Here's how the part is built. I have some questions about the finished solid (model axes, mm). Coordinates: 2 decimals unless noted, no trailing zeros. Write each loop counter-clockwise with the first axis right and the second up, starting at its lowest first coordinate (ties: lowest second). Pieces come first, ordered by that corner, then holes. Notation, with made-up numbers: (-30, 44) -> (15, 44) arc R19 ccw to (15, 79) -> close; hole circle Ø8 at (-38, 3.5). An arc over 180 degrees is marked (long way). Put each result on its own line as item: value. Start each with the question number.
Item 1: I need wall thicknesses on line 1 (X direction, y = -1, z = -1); line 2 (Z direction, x = 2, y = -0.05); line 3 (Z direction, x = -2, y = -0.9). Which ranges of each line are inside material? Lowest first, please. Write a range as [from, to].
Item 2: For pin 1 (0.9 mm diameter, centred on y = -0.5, z = 0.5, fed in from -X), with a flat end and sliding along its axis, tell me the tip position at first contact or that it passes through.
Item 3: I want a section at C-C, the plane z = 0.15. List the corners of the cut face in (x, y) for me, then the cut area to 3 significant figures.
Item 4: I want a section at D-D, the plane x = 0.25. List the corners of the cut face in (y, z) for me, then the cut area to 3 significant figures.
Item 5: If we mould it in two halves opening along Z, with no side actions, what happens to faces 1 (the face through (0, 0.4, 0)), 2 (the face through (-1, -0.25, 0)), 3 (the face through (-0.51, 0.07, -1.5)), 4 (the face through (-1, 0.25, 0))? For each: released by +Z, released by -Z, zero draft, split by the parting line, or undercut.
Item 6: I want a section at B-B, the plane y = -0.15. List the corners of the cut face in (x, z) for me.
Autodesk Inventor part; units mm, degrees
ref_plane "YZ Plane" through (0, 0, 0) normal (1, 0, 0) x (0, 1, 0)
ref_plane "XZ Plane" through (0, 0, 0) normal (0, 1, 0) x (-1, 0, 0)
ref_plane "XY Plane" through (0, 0, 0) normal (0, 0, 1) x (1, 0, 0)
sketch "Body" plane through (0, 0, 0) normal (0, 1, 0) x (-1, 0, 0)
  line L0 (0, 1.5) -> (0, 0)
  line L1 (0, 1.5) -> (1, 1.5)
  line L2 (1, 1.5) -> (1, 1.25)
  line L3 (0, 0) -> (4.2, 0)
  arc A0 (4.2, 0) -> (2.95, 1.25) centre (2.95, 0) ccw
  line L4 (2.95, 1.25) -> (1, 1.25)
  point P0 (0, 0)
  dimension "d1" = 1
  dimension "d2" = 4.2
  dimension "d3" = 1.5
  dimension "d4" = 0.25
revolve "Revolution1" add sketch "Body" angle 360 about axis through (0, 0, 0) along (-1, 0, 0)
sketch "Sketch2" plane through (0, 0, 0) normal (1, 0, 0) x (0, 0, -1)
  line L0 (-1, 0.25) -> (1, 0.25)
  line L1 (1, 0.25) -> (1, -0.25)
  line L2 (1, -0.25) -> (-1, -0.25)
  line L3 (-1, -0.25) -> (-1, 0.25)
  circle A0 centre (0, 0) radius 1.5 construction
  line L4 (-1, 0) -> (1, 0) construction
  dimension "d9" = 0.5
  dimension "d10" = 0.5
extrude "Extrusion1" cut sketch "Sketch2" against normal blind 2.25
sketch "Sketch3" plane through (-2.25, 0, 0) normal (1, 0, 0) x (0, 0, -1)
  circle A0 centre (-0.75, 0) radius 0.25
  line L0 (-1, 0.25) -> (1, 0.25) construction
  line L1 (1, -0.25) -> (-1, -0.25) construction
  line L2 (-1, -0.25) -> (-1, 0.25)
  line L3 (0, 0.25) -> (0, -0.25) construction
  circle A1 centre (0.75, 0) radius 0.25
  point P0 (0, 0)
extrude "Extrusion2" add sketch "Sketch3" along normal blind 5
properties part number "Led3mm"
Calculated:
1. line 1: x = [-1, 0]
1. line 2: z = [-0.99, -0.51], [0.51, 0.99]
1. line 3: z = [-0.87, 0.87]
2. pin 1: stops at x = -4.17
3. outline: (-2.95, -1.24) -> (-1, -1.24) -> (-1, -1.49) -> (0, -1.49) -> (0, -0.25) -> (-2.25, -0.25) -> (-2.25, 0.25) -> (0, 0.25) -> (0, 1.49) -> (-1, 1.49) -> (-1, 1.24) -> (-2.95, 1.24) arc R1.24 ccw to start
3. area: 9.12 mm2
4. outline: circle Ø0.5 at (0, -0.75); circle Ø0.5 at (0, 0.75)
4. area: 0.393 mm2
5. face 1: zero draft
5. face 2: undercut
5. face 3: split by the parting line
5. face 4: undercut
6. outline: (-2.95, -1.24) -> (-1, -1.24) -> (-1, -1.49) -> (0, -1.49) -> (0, -1) -> (-2.25, -1) -> (-2.25, -0.95) -> (2.75, -0.95) -> (2.75, -0.55) -> (-2.25, -0.55) -> (-2.25, 0.55) -> (2.75, 0.55) -> (2.75, 0.95) -> (-2.25, 0.95) -> (-2.25, 1) -> (0, 1) -> (0, 1.49) -> (-1, 1.49) -> (-1, 1.24) -> (-2.95, 1.24) arc R1.24 ccw to start
